The drawing under review shows one solid part. Ordinate dimensions are in mm from its lowest x, y, z. Round coordinates to 2 decimals unless told otherwise and drop trailing zeros. Order: outer loops, then holes, each group sorted by start corner. A loop starts at its lowest first (then second) coordinate and runs counter-clockwise, first axis right, second up. Notation, with made-up numbers: M 50,5 L 57,5 A26 cw 57,38 Z; hole C -25,39.25 d10. An arc over 180 degrees is marked long. Answer as a JSON object with one key per item and string values. Group by question number.
1) Consider section C-C, the plane y = 72. Write out the cut boundary in (x, z).
2) The part is to be moulded in two halves that separate along Z. For the marked faces 1 and 2, say which applies: +Z half, -Z half, draft (parallel to the pull), parting line (faces both ways), or undercut.
3) Consider section A-A, the plane z = 49. Write out the cut boundary in (x, y).
4) Consider section B-B, the plane x = 1.25. Write out the cut boundary in (y, z).
5) Insertion check: pin 1 Ø0.9 at (x, z) = (2, 50) entering from +Y; pin 2 Ø8 at (y, z) = (87.5, 65) entering from +X; pin 3 Ø12 at (y, z) = (76, 75) entering from -X. Each pin has a flat end and moves straight along its axis. Give the tip position at first contact, or say it passes through.
6) To check wall thickness, follow line 1 (Y direction, x = 6.5, z = 49); line 2 (X direction, y = 85, z = 51); line 3 (Y direction, x = 4.75, z = 31). State the ranges of each line that lie inside material, in increasing order.
7) Consider section D-D, the plane y = 31. Write out the cut boundary in (x, z).
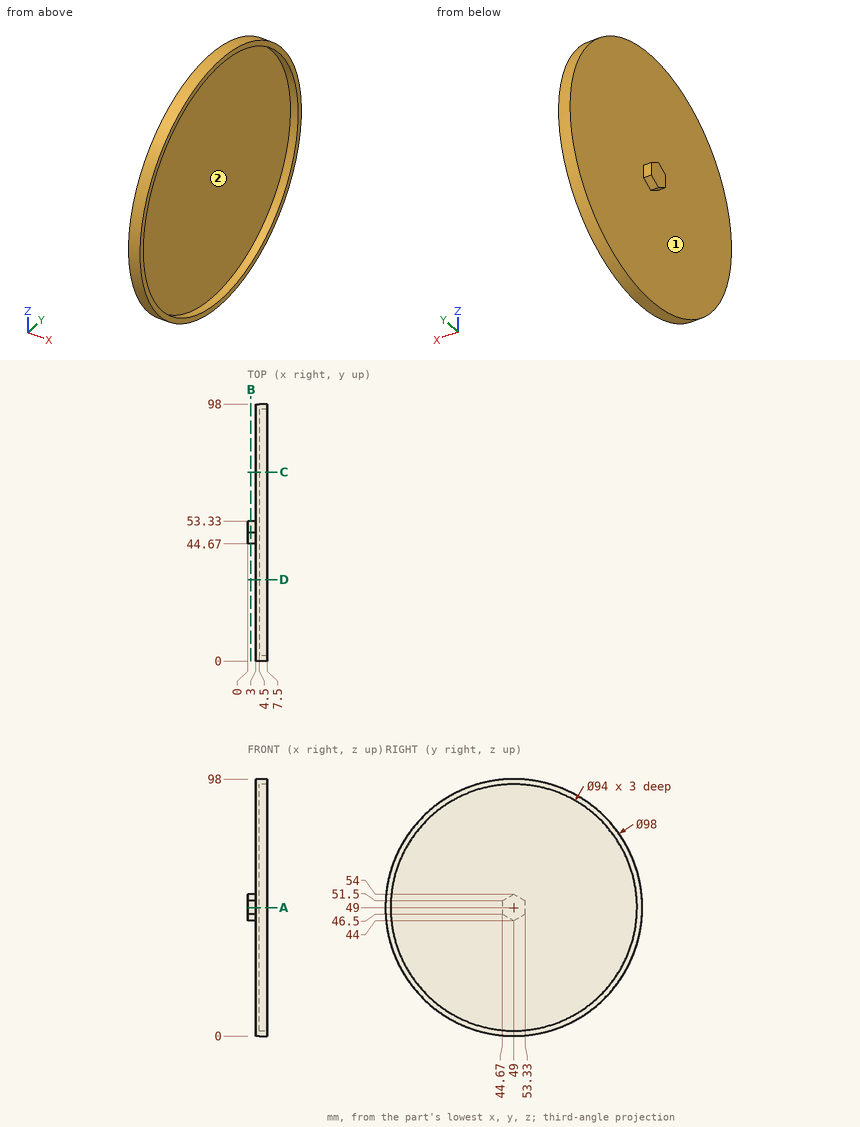
Results list:
{
 "1": {"outline": "M 3,5.73 L 7.5,5.73 L 7.5,8.01 L 4.5,8.01 L 4.5,89.99 L 7.5,89.99 L 7.5,92.27 L 3,92.27 Z"},
 "2": {"face 1": "draft", "face 2": "undercut"},
 "3": {"outline": "M 0,44.67 L 3,44.67 L 3,0 L 7.5,0 L 7.5,2 L 4.5,2 L 4.5,96 L 7.5,96 L 7.5,98 L 3,98 L 3,53.33 L 0,53.33 Z"},
 "4": {"outline": "M 44.67,46.5 L 49,44 L 53.33,46.5 L 53.33,51.5 L 49,54 L 44.67,51.5 Z"},
 "5": {"pin 1": "y = 53.33", "pin 2": "x = 4.5", "pin 3": "x = 3"},
 "6": {"line 1": "0 to 2, 96 to 98", "line 2": "3 to 4.5", "line 3": "3.43 to 5.58, 92.42 to 94.57"},
 "7": {"outline": "M 3,3.43 L 7.5,3.43 L 7.5,5.58 L 4.5,5.58 L 4.5,92.42 L 7.5,92.42 L 7.5,94.57 L 3,94.57 Z"}
}
